```python
from build123d import *

# Parameters (mm, degrees)
F1_DEPTH = 10
F3_DEPTH = 2
F5_DEPTH = 1


with BuildPart() as f1:
    # F0 (on Top) → F1 (new body)
    with BuildSketch(Plane.XY):
        with BuildLine():
            ThreePointArc((57, 32), (0, 89), (-57, 32))
            Line((-57, 32), (-57, -32))
            ThreePointArc((-57, -32), (0, -89), (57, -32))
            Line((57, -32), (57, 32))
        make_face()
        with BuildLine():
            ThreePointArc((-46, 32), (0, 78), (46, 32))
            Line((46, 32), (46, -32))
            ThreePointArc((46, -32), (0, -78), (-46, -32))
            Line((-46, -32), (-46, 32))
        make_face(mode=Mode.SUBTRACT)
    extrude(amount=F1_DEPTH)

    # F2 (on face) → F3 (cut)
    with BuildSketch(Plane(origin=(0, 0, 0), x_dir=(1, 0, 0), z_dir=(0, 0, -1))):
        with BuildLine():
            ThreePointArc((55, 32), (0, 87), (-55, 32))
            Line((-55, 32), (-55, -32))
            ThreePointArc((-55, -32), (0, -87), (55, -32))
            Line((55, -32), (55, 32))
        make_face()
        with BuildLine():
            Line((-48, -32), (-48, 32))
            ThreePointArc((-48, 32), (0, 80), (48, 32))
            Line((48, 32), (48, -32))
            ThreePointArc((48, -32), (0, -80), (-48, -32))
        make_face(mode=Mode.SUBTRACT)
    extrude(amount=-F3_DEPTH, mode=Mode.SUBTRACT)

    # F4 (on face) → F5 (cut)
    with BuildSketch(Plane(origin=(0, 0, 2), x_dir=(1, 0, 0), z_dir=(0, 0, -1))):
        with BuildLine():
            Line((52.5, 10), (52.5, 32))
            ThreePointArc((52.5, 32), (0, 84.5), (-52.5, 32))
            Line((-52.5, 32), (-52.5, 10))
            Line((-52.5, 10), (-50.5, 10))
            Line((-50.5, 10), (-50.5, 32))
            ThreePointArc((-50.5, 32), (0, 82.5), (50.5, 32))
            Line((50.5, 32), (50.5, 10))
            Line((50.5, 10), (52.5, 10))
        make_face()
        with BuildLine():
            Line((-52.5, -10), (-52.5, -32))
            ThreePointArc((-52.5, -32), (0, -84.5), (52.5, -32))
            Line((52.5, -32), (52.5, -10))
            Line((52.5, -10), (50.5, -10))
            Line((50.5, -10), (50.5, -32))
            ThreePointArc((50.5, -32), (0, -82.5), (-50.5, -32))
            Line((-50.5, -32), (-50.5, -10))
            Line((-50.5, -10), (-52.5, -10))
        make_face()
    extrude(amount=-F5_DEPTH, mode=Mode.SUBTRACT)


solid = f1.part
```
Design review of the part built by this model. Coordinates are the model's own, in mm. A direction names the side the tool comes from. Round coordinates to 2 decimals unless told otherwise and drop trailing zeros. Write each loop counter-clockwise with the first axis right and the second up, starting at its lowest first coordinate (ties: lowest second). Pieces come first, ordered by that corner, then holes.
Item 1: We need section B-B on z = 5.5. Write out the cut boundary in (x, y), and give its area (3 significant figures).
Item 2: Clearance check with flat-ended pins moving along their axes: pin 1 Ø1.5 at (x, z) = (21, 3.5) entering from -Y; pin 2 Ø3 at (x, z) = (-23.5, 3) entering from -Y; pin 3 Ø0.8 at (x, z) = (-51.5, 2.5) entering from -Y. State where each tip first meets the part, or that it passes through.
Item 3: We need section C-C on x = 0. Write out the cut boundary in (y, z).
Item 4: For probe 1 along X at (y, z) = (-45.5, 2.25); probe 2 along X at (y, z) = (27, 8); probe 3 along Y at (x, z) = (36.5, 1), list the stretches that pass through material, from the lowest coordinate up.
Item 5: For faces 4 (the flat face through (57, 0, 5)), 5 (the cylindrical face through (-1.06, -79.99, 0.99)), 6 (the cylindrical face through (-1.01, 77.99, 4.93)), list the 3-axis set-ups (+Z, -Z, +X, -X, +Y, -Y) from which the entire face can be reached by the end or side of a thin tool; tool diameter is ignored.
Item 6: The part is to be moulded in two halves that separate along Y. For faces 1 (the cylindrical face through (-1.253, -88.986, 4.93)), 2 (the flat face through (46, 0, 5)), 3 (the flat face through (-47, 0, 10)), say which applies: +Y half, -Y half, draft (parallel to the pull), parting line (faces both ways), or undercut.
Item 7: We need section A-A on y = 7. Write out the cut boundary in (x, z), and give its area (3 significant figures).
Item 8: We need section D-D on y = -22. Write out the cut boundary in (x, z).
Returned:
1. outline: (-57, -32) arc R57 ccw to (57, -32) - (57, 32) arc R57 ccw to (-57, 32) - close; hole (-46, -32) arc R46 ccw to (46, -32) - (46, 32) arc R46 ccw to (-46, 32) - close
1. area: 4,970 mm2
2. pin 1: stops at y = -85.28
2. pin 2: stops at y = -84.58
2. pin 3: stops at y = -57.25
3. outline: (-89, 0) - (-87, 0) - (-87, 2) - (-84.5, 2) - (-84.5, 3) - (-82.5, 3) - (-82.5, 2) - (-80, 2) - (-80, 0) - (-78, 0) - (-78, 10) - (-89, 10) - close; (78, 0) - (80, 0) - (80, 2) - (82.5, 2) - (82.5, 3) - (84.5, 3) - (84.5, 2) - (87, 2) - (87, 0) - (89, 0) - (89, 10) - (78, 10) - close
4. probe 1: x = -55.38 to -50.73, -48.66 to -43.97, 43.97 to 48.66, 50.73 to 55.38
4. probe 2: x = -57 to -46, 46 to 57
4. probe 3: y = -75.78 to -73.14, -63.17 to -60, 60 to 63.17, 73.14 to 75.78
5. face 4: +Z, -Z, +X, +Y, -Y
5. face 5: -Z
5. face 6: +Z, -Z
6. face 1: -Y half
6. face 2: undercut
6. face 3: draft
7. outline: (-57, 0) - (-55, 0) - (-55, 2) - (-48, 2) - (-48, 0) - (-46, 0) - (-46, 10) - (-57, 10) - close; (46, 0) - (48, 0) - (48, 2) - (55, 2) - (55, 0) - (57, 0) - (57, 10) - (46, 10) - close
7. area: 192 mm2
8. outline: (-57, 0) - (-55, 0) - (-55, 2) - (-52.5, 2) - (-52.5, 3) - (-50.5, 3) - (-50.5, 2) - (-48, 2) - (-48, 0) - (-46, 0) - (-46, 10) - (-57, 10) - close; (46, 0) - (48, 0) - (48, 2) - (50.5, 2) - (50.5, 3) - (52.5, 3) - (52.5, 2) - (55, 2) - (55, 0) - (57, 0) - (57, 10) - (46, 10) - close
